```python
from build123d import *

# Parameters (mm, degrees)
SKETCH1_R           = 2.25
SKETCH1_R_2         = 44.958
SKETCH1_R_3         = 1.65
SKETCH1_R_4         = 1.5
BOSS_EXTRUDE1_DEPTH = 5.842
SKETCH2_R           = 44.958
SKETCH2_R_2         = 43
BOSS_EXTRUDE2_DEPTH = 5.842
SKETCH3_W           = 42
SKETCH3_H           = 6.35
CUT_EXTRUDE1_DEPTH  = 78.066295668
SKETCH4_R           = 0.5
CUT_EXTRUDE2_DEPTH  = 78.066295668
FILLET1_R           = 3


with BuildPart() as part:
    # Sketch1 → Boss-Extrude1 (new body)
    with BuildSketch(Plane.XY):
        with BuildLine():
            Line((-50.8, 0), (-50.8, -57.658))
            Line((-50.8, -57.658), (50.8, -57.658))
            Line((50.8, -57.658), (50.8, 0))
            ThreePointArc((50.8, 0), (0, 50.8), (-50.8, 0))
        make_face()
        with Locations((41.8, -47.658)):
            Circle(SKETCH1_R, mode=Mode.SUBTRACT)
        Circle(SKETCH1_R_2, mode=Mode.SUBTRACT)
        with Locations((-47.879, 0)):
            Circle(SKETCH1_R_3, mode=Mode.SUBTRACT)
        with Locations((0, 47.879)):
            Circle(SKETCH1_R_3, mode=Mode.SUBTRACT)
        with Locations((41.8, -27.658)):
            Circle(SKETCH1_R, mode=Mode.SUBTRACT)
        with Locations((47.879, 0)):
            Circle(SKETCH1_R_3, mode=Mode.SUBTRACT)
        with Locations((0, -47.879)):
            Circle(SKETCH1_R_3, mode=Mode.SUBTRACT)
        with Locations((-33.855565576, 33.855565576)):
            Circle(SKETCH1_R_4, mode=Mode.SUBTRACT)
        with Locations((33.855565576, 33.855565576)):
            Circle(SKETCH1_R_4, mode=Mode.SUBTRACT)
        with Locations((33.855565576, -33.855565576)):
            Circle(SKETCH1_R_4, mode=Mode.SUBTRACT)
        with Locations((-33.855565576, -33.855565576)):
            Circle(SKETCH1_R_4, mode=Mode.SUBTRACT)
        with Locations((-41.8, -27.658)):
            Circle(SKETCH1_R, mode=Mode.SUBTRACT)
        with Locations((-41.8, -47.658)):
            Circle(SKETCH1_R, mode=Mode.SUBTRACT)
    extrude(amount=BOSS_EXTRUDE1_DEPTH)

    # Sketch2 → Boss-Extrude2 (add, through all)
    with BuildSketch(Plane.XY.offset(5.842)):
        Circle(SKETCH2_R)
        Circle(SKETCH2_R_2, mode=Mode.SUBTRACT)
    extrude(amount=-BOSS_EXTRUDE2_DEPTH)

    # Sketch3 → Cut-Extrude1 (cut, through all)
    with BuildSketch(Plane.XY.offset(5.842)):
        with Locations((0, -54.483)):
            Rectangle(SKETCH3_W, SKETCH3_H)
    extrude(amount=-CUT_EXTRUDE1_DEPTH, mode=Mode.SUBTRACT)

    # Sketch4 → Cut-Extrude2 (cut, through all)
    with BuildSketch(Plane.XY.offset(5.842)):
        with Locations((-21, -51.308)):
            Circle(SKETCH4_R)
        with Locations((21, -51.308)):
            Circle(SKETCH4_R)
    extrude(amount=-CUT_EXTRUDE2_DEPTH, mode=Mode.SUBTRACT)

    # Fillet1
    fillet1_edges = [part.edges().sort_by_distance(p)[0] for p in [
        (50.8, -57.658, 2.921),
        (-50.8, -57.658, 2.921),
        (-21, -57.658, 2.921),
        (21, -57.658, 2.921),
    ]]
    fillet(fillet1_edges, radius=FILLET1_R)


solid = part.part
```
Here's how the part is built. I have some questions about the finished solid (model axes, mm). A direction names the side the tool comes from. Give positions to 0.01 mm unless a question says otherwise; leave off trailing zeros. Write each loop counter-clockwise with the first axis right and the second up, starting at its lowest first coordinate (ties: lowest second). Pieces come first, ordered by that corner, then holes. Notation, with made-up numbers: (41.25, 30) -> (47.25, 30) arc R12 cw to (47.25, 41) -> close; hole circle Ø6 at (19.5, 25). An arc over 180 degrees is marked (long way). Use one line per item in the form item = value.
1) Suppose I cut it at B-B (x = -10.5). Please give me the cut outline in (y, z).
Verdict:
outline = (-51.31, 0) -> (-41.7, 0) -> (-41.7, 5.84) -> (-51.31, 5.84) -> close; (41.7, 0) -> (49.7, 0) -> (49.7, 5.84) -> (41.7, 5.84) -> close
2) Suppose I cut it at C-C (y = 10.5). Please give me the cut outline in (x, z).
Verdict:
outline = (-49.7, 0) -> (-41.7, 0) -> (-41.7, 5.84) -> (-49.7, 5.84) -> close; (41.7, 0) -> (49.7, 0) -> (49.7, 5.84) -> (41.7, 5.84) -> close
3) I'm going to push flat-ended pins straight in: pin 1 (3 mm diameter, centred on x = -2.5, z = 1.5, fed in from -Y); pin 2 (3 mm diameter, centred on x = 0, y = 47.879, fed in from +Z). Where does each tip first touch, or does it pass through?
Verdict:
pin_1 = -51.31
pin_2 = through
4) We'd pull the mould along Y, two halves only. Please class faces 3 (the face through (1.117, 50.788, 2.88)), 4 (the face through (21, -53, 3)), 5 (the face through (41.312, -49.854, 2.88)): +Y half, -Y half, draft (parallel to the pull), parting line (faces both ways), or undercut.
Verdict:
face_3 = +Y half
face_4 = draft
face_5 = undercut
5) If I drill on L1, parallel to Y at x = 0, z = 4.25; L2, parallel to X at y = -26, z = 4.05; L3, parallel to Y at x = -32.5, z = 4, over which ranges is the centre line in solid material (lowest first)? Write a range as [from, to].
Verdict:
L1 = [-51.31, -49.53], [-46.23, -43], [43, 46.23], [49.53, 50.8]
L2 = [-50.8, -43.32], [-40.28, -34.25], [34.25, 40.28], [43.32, 50.8]
L3 = [-57.66, -34.5], [-33.21, -28.16], [28.16, 33.21], [34.5, 39.04]
6) Suppose I cut it at A-A (x = 0). Please give me the cut outline in (y, z).
Verdict:
outline = (-51.31, 0) -> (-49.53, 0) -> (-49.53, 5.84) -> (-51.31, 5.84) -> close; (-46.23, 0) -> (-43, 0) -> (-43, 5.84) -> (-46.23, 5.84) -> close; (43, 0) -> (46.23, 0) -> (46.23, 5.84) -> (43, 5.84) -> close; (49.53, 0) -> (50.8, 0) -> (50.8, 5.84) -> (49.53, 5.84) -> close
7) On a 3-axis mill with a long thin cutter (end or side, diameter ignored), from which of +Z, -Z, +X, -X, +Y, -Y can I reach the whole of each face in a straight line? I mean faces 1 (the face through (-21, -53, 3)), 2 (the face through (-35.354, 33.922, 2.88)). Say none if no direction works.
Verdict:
face_1 = +Z, -Z, -Y
face_2 = +Z, -Z
8) Suppose I cut it at D-D (z = 4.2). Give the number of separate pieces and of enclosed holes in the cut face, and give its area (3 significant figures).
Verdict:
separate_pieces = 1
enclosed_holes = 13
area = 3,700 mm2
